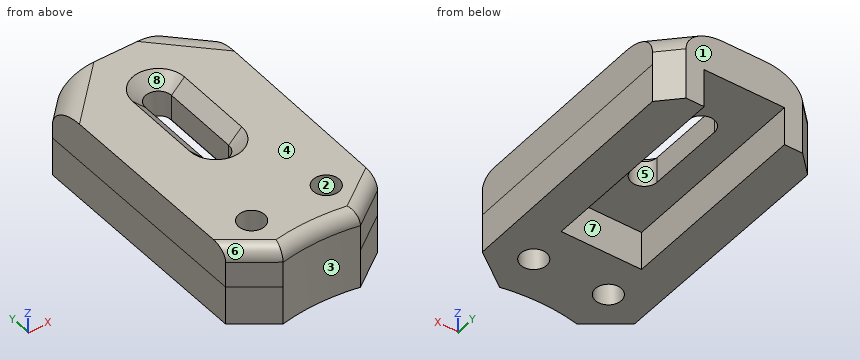
Autodesk Inventor part; units mm, degrees
ref_plane "YZ Plane" through (0, 0, 0) normal (1, 0, 0) x (0, 1, 0)
ref_plane "XZ Plane" through (0, 0, 0) normal (0, 1, 0) x (-1, 0, 0)
ref_plane "XY Plane" through (0, 0, 0) normal (0, 0, 1) x (1, 0, 0)
sketch "Sketch1" plane through (0, 0, 0) normal (0, 0, 1) x (1, 0, 0)
  circle A0 centre (2.8817, -5.5305) radius 1
  circle A1 centre (-2.8817, -5.5305) radius 1
  line L0 (4.5, 12.6443) -> (5.9902, 11.1443)
  line L1 (3, 12.6443) -> (4.5, 12.6443)
  line L2 (3, -2.3557) -> (3, 12.6443)
  line L3 (-3, -2.3557) -> (3, -2.3557)
  line L4 (-3, 12.6443) -> (-3, -2.3557)
  line L5 (-4.5, 12.6443) -> (-3, 12.6443)
  line L6 (-5.9902, 11.1443) -> (-4.5, 12.6443)
  line L7 (-5.8406, -11.8556) -> (-5.9902, 11.1443)
  line L8 (-3.8536, -9.8557) -> (-5.8406, -11.8556)
  line L9 (-3.8536, -9.8557) -> (3.8536, -9.8557)
  line L10 (5.8406, -11.8556) -> (3.8536, -9.8557)
  line L11 (5.9902, 11.1443) -> (5.8406, -11.8556)
  line L12 (3.8536, -9.8557) -> (5.8536, -9.8557)
  line L13 (-3.8536, -9.8557) -> (-5.8535, -9.8687)
  point P0 (0, 0)
extrude "Extrusion1" add sketch "Sketch1" along normal blind 3 contours L0 L11 L12 L9 L13 L7 L6 L5 L4 L3 L2 L1
sketch "Sketch2" plane through (0, 0, 3) normal (0, 0, 1) x (1, 0, 0)
  line L0 (-3, -2.3557) -> (-3, 12.6443)
  line L1 (-3, 12.6443) -> (-4.5, 12.6443)
  line L2 (-4.5, 12.6443) -> (-5.9902, 11.1443)
  line L3 (-5.9902, 11.1443) -> (-5.8535, -9.8687)
  line L4 (-5.8535, -9.8687) -> (-3.8536, -9.8557)
  line L5 (-3.8536, -9.8557) -> (5.8536, -9.8557)
  line L6 (5.8536, -9.8557) -> (5.9902, 11.1443)
  line L7 (5.9902, 11.1443) -> (4.5, 12.6443)
  line L8 (4.5, 12.6443) -> (3, 12.6443)
  line L9 (3, 12.6443) -> (3, -2.3557)
  line L10 (3, -2.3557) -> (-3, -2.3557)
  circle A0 centre (-2.8817, -5.5305) radius 1
  circle A1 centre (2.8817, -5.5305) radius 1
  line L11 (3, 12.6443) -> (3, -2.3557)
  line L12 (-3, 12.6443) -> (3, 12.6443)
  point P0 (0, 0)
extrude "Extrusion2" add sketch "Sketch2" along normal blind 3
sketch "Sketch3" plane through (0, 0, 6) normal (0, 0, 1) x (1, 0, 0)
  line L0 (-5.8535, -9.8687) -> (-3.8536, -9.8557)
  line L1 (-3.8536, -9.8557) -> (5.8536, -9.8557)
  line L2 (5.8536, -9.8557) -> (5.9902, 11.1443)
  line L3 (5.9902, 11.1443) -> (4.5, 12.6443)
  line L4 (4.5, 12.6443) -> (-4.5, 12.6443)
  line L5 (-4.5, 12.6443) -> (-5.9902, 11.1443)
  line L6 (-5.9902, 11.1443) -> (-5.8535, -9.8687)
  circle A0 centre (2.8817, -5.5305) radius 1
  circle A1 centre (-2.8817, -5.5305) radius 1
  line L7 (-5.8535, -9.8687) -> (-3.8536, -9.8557)
  arc A2 (5.8536, -9.8557) -> (-5.8535, -9.8687) centre (0.0154, -23.6729) ccw
  point P0 (0, 0)
  dimension "d4" = 15
extrude "Extrusion3" cut sketch "Sketch3" against normal blind 8 contours A2 L1 L0
chamfer "Chamfer1" distance 3 angle 45 2 edges at (5.8536, -9.8557, 3) (-5.8535, -9.8687, 3)
fillet "Fillet1" radius 2 2 edges at (5.2451, 11.8943, 6) (-5.2451, 11.8943, 6)
fillet "Fillet2" radius 1 3 edges at (-4.4311, -7.9228, 6) (-0.0013, -8.6729, 6) (4.4302, -7.913, 6)
sketch "Sketch4" plane through (0, 0, 6) normal (0, 0, 1) x (1, 0, 0)
  line L0 (-1, 8.1443) -> (-1, 2.1443)
  arc A0 (-1, 2.1443) -> (1, 2.1443) centre (0, 2.1443) ccw
  line L1 (1, 2.1443) -> (1, 8.1443)
  arc A1 (1, 8.1443) -> (-1, 8.1443) centre (0, 8.1443) ccw
  line L2 (5.9719, 8.3251) -> (1.6807, 12.6443)
  line L3 (5.9719, 8.3251) -> (5.8537, -9.8477)
  line L4 (3.4979, -11.4182) -> (5.8537, -9.8477)
  spline S0 degree 3 poles (3.7471, -14.0453) (3.5143, -13.7817) (3.313, -13.4738) (3.0785, -12.9028) (3.0205, -12.6553) (3.011, -12.2509) (3.0346, -12.0815) (3.1344, -11.8203) (3.188, -11.725) (3.325, -11.5531) (3.4063, -11.4793) (3.4979, -11.4182) knots 0 0 0 0 0.329568 0.329568 0.580897 0.580897 0.763488 0.763488 0.881593 0.881593 1 1 1 1
  arc A2 (-3.7471, -14.0453) -> (3.7471, -14.0453) centre (0, -17.3557) ccw
  spline S1 degree 3 poles (-3.4979, -11.4182) (-3.3811, -11.4961) (-3.2816, -11.5944) (-3.1273, -11.8263) (-3.0754, -11.9539) (-3.0096, -12.2519) (-3.0068, -12.4209) (-3.0565, -12.825) (-3.1338, -13.0604) (-3.3668, -13.5541) (-3.5446, -13.816) (-3.7471, -14.0453) knots 0 0 0 0 0.142201 0.142201 0.282073 0.282073 0.450832 0.450832 0.692964 0.692964 1 1 1 1
  line L5 (-5.8537, -9.8477) -> (-3.4979, -11.4182)
  line L6 (-5.8537, -9.8477) -> (-5.9719, 8.3251)
  line L7 (-1.6807, 12.6443) -> (-5.9719, 8.3251)
  line L8 (-1.6807, 12.6443) -> (1.6807, 12.6443)
  circle A3 centre (0, -17.3557) radius 1.5
  circle A4 centre (-2.8817, -5.5305) radius 1
  circle A5 centre (2.8817, -5.5305) radius 1
  point P0 (0, 0)
extrude "Extrusion4" cut sketch "Sketch4" against normal blind 8 contours A1 L1 A0 L0
chamfer "Chamfer2" distance 1 angle 45 4 edges at (-1, 5.1443, 6) (0, 9.1443, 6) (1, 5.1443, 6) (0, 1.1443, 6)
thicken "Thicken1" operation add thickness 0.1 both sides no extend neighbours yes toward (-1, 0, 0) faces at (-3, 2.6443, 1)
thicken "Thicken2" operation add thickness 0.1 both sides no extend neighbours yes toward (1, 0, 0) faces at (3, 7.6443, 1)
properties part number "arm_linkage_3"
Geometry check sheet. Reference: the model listing, model coordinates, mm. Face numbers are marked on the shaded views. A direction names the side the tool comes from. Round coordinates to 2 decimals unless told otherwise and drop trailing zeros. Order: outer loops, then holes, each group sorted by start corner. A loop starts at its lowest first (then second) coordinate and runs counter-clockwise, first axis right, second up. Notation, with made-up numbers: M 78,2 L 103,2 A22 cw 103,38 Z; hole C 66.5,-24 d4. An arc over 180 degrees is marked long. Answer in a Markdown table with one row per item.
(1) Draft check along Y on the marked faces 1, 2 and 3. Enter one of: released by +Y, released by -Y, zero draft, split by the parting line, or undercut.
Responses:
| item | result |
|---|---|
| face 1 | released by +Y |
| face 2 | undercut |
| face 3 | released by -Y |
(2) Sectioned sample at C-C, the plane z = 2. Record the cut outline in (x, y).
Responses:
| item | result |
|---|---|
| outline | M -5.99,11.14 L -5.87,-6.87 L -2.99,-8.98 A15 cw 2.99,-8.97 L 5.87,-6.86 L 5.99,11.14 L 4.5,12.64 L 3.1,12.64 L 3.1,-2.36 L -3.1,-2.36 L -3.1,12.64 L -4.5,12.64 Z; hole C -2.88,-5.53 d2; hole C 2.88,-5.53 d2 |
(3) Sectioned sample at A-A, the plane y = 7. Record the cut outline in (x, z).
Responses:
| item | result |
|---|---|
| outline | M -5.96,0 L -3.1,0 L -3.1,3 L -1,3 L -1,5 L -2,6 L -5.96,6 Z; M 1,3 L 3.1,3 L 3.1,0 L 5.96,0 L 5.96,6 L 2,6 L 1,5 Z |
(4) Scan lines: probe 1 along X at (y, z) = (-5.5, 4.25); probe 2 along X at (y, z) = (7.5, 1.75); probe 3 along Z at (x, y) = (2.25, 6.25). Record each from-to range of solid material in increasing order. Write a range as from..to.
Responses:
| item | result |
|---|---|
| probe 1 | x = -5.88..-3.88, -1.88..1.88, 3.88..5.88 |
| probe 2 | x = -5.97..-3.1, 3.1..5.97 |
| probe 3 | z = 3..6 |
(5) Sectioned sample at B-B, the plane z = 5.25. Record the cut outline in (x, y).
Responses:
| item | result |
|---|---|
| outline | M -5.99,10.53 L -5.87,-6.83 L -2.98,-8.94 A15.03 cw 2.98,-8.94 L 5.87,-6.82 L 5.99,10.53 L 3.88,12.64 L -3.88,12.64 Z; hole C -2.88,-5.53 d2; hole M -1.25,2.14 A1.25 ccw 1.25,2.14 L 1.25,8.14 A1.25 ccw -1.25,8.14 Z; hole C 2.88,-5.53 d2 |
(6) Sectioned sample at D-D, the plane z = 4.25. Record the cut outline in (x, y).
Responses:
| item | result |
|---|---|
| outline | M -5.99,11.12 L -5.87,-6.87 L -2.99,-8.98 A15 cw 2.99,-8.97 L 5.87,-6.86 L 5.99,11.12 L 4.48,12.64 L -4.48,12.64 Z; hole C -2.88,-5.53 d2; hole M -1,2.14 A1 ccw 1,2.14 L 1,8.14 A1 ccw -1,8.14 Z; hole C 2.88,-5.53 d2 |
(7) Go/stop test with flat-tipped pins: P1, Ø0.9, axis at x = 0.5, z = 1.5, coming from the +Y side; P2, Ø1, axis at x = -1, z = 3.5, coming from the -Y side; P3, Ø1, axis at x = -1, y = -1.5, coming from the -Z side. Record where each tip stops, or that it passes through.
Responses:
| item | result |
|---|---|
| P1 | stops at y = -2.36 |
| P2 | stops at y = -8.75 |
| P3 | stops at z = 3 |
(8) Tool access check on the marked faces 4, 5, 6, 7 and 8. Record the directions out of +Z, -Z, +X, -X, +Y, -Y that give a thin tool (end or side, any length) a straight path to the whole face; none if there is none.
Responses:
| item | result |
|---|---|
| face 4 | +Z, +X, -X, +Y, -Y |
| face 5 | +Z, -Z |
| face 6 | +Z, -X, -Y |
| face 7 | -Z, +Y |
| face 8 | +Z |
